from build123d import *

# Parameters (mm, degrees)
ESQUISSE1_W             = 24
ESQUISSE1_H             = 22
BOSS_EXTRU_1_DEPTH      = 2
ENL_V_MAT_EXTRU_1_DEPTH = 2
ESQUISSE3_R             = 1.75
ENL_V_MAT_EXTRU_2_DEPTH = 2
ESQUISSE4_R             = 2.894655209
ENL_V_MAT_EXTRU_3_DEPTH = 2
BOSS_EXTRU_2_DEPTH      = 10
ESQUISSE6_W             = 10
ESQUISSE6_H             = 10
ENL_V_MAT_EXTRU_4_DEPTH = 10
BOSS_EXTRU_3_DEPTH      = 2


with BuildPart() as part:
    # Esquisse1 → Boss.-Extru.1 (new body)
    with BuildSketch(Plane(origin=(0, 0, 0), x_dir=(1, 0, 0), z_dir=(0, 1, 0))):
        with Locations((12, 11)):
            Rectangle(ESQUISSE1_W, ESQUISSE1_H)
    extrude(amount=BOSS_EXTRU_1_DEPTH)

    # Esquisse2 → Enlèv. mat.-Extru.1 (cut)
    with BuildSketch(Plane(origin=(0, 2, 0), x_dir=(1, 0, 0), z_dir=(0, 1, 0))):
        Polygon((1, 21), (23, 21), (23, 10), (13, 10), (13, 1), (1, 1), align=None)
    extrude(amount=-ENL_V_MAT_EXTRU_1_DEPTH, mode=Mode.SUBTRACT)

    # Esquisse3 → Enlèv. mat.-Extru.2 (cut)
    with BuildSketch(Plane(origin=(0, 2, 0), x_dir=(1, 0, 0), z_dir=(0, 1, 0))):
        with Locations((18.75, 5)):
            Circle(ESQUISSE3_R)
    extrude(amount=-ENL_V_MAT_EXTRU_2_DEPTH, mode=Mode.SUBTRACT)

    # Esquisse4 → Enlèv. mat.-Extru.3 (cut)
    with BuildSketch(Plane(origin=(0, 2, 0), x_dir=(1, 0, 0), z_dir=(0, 1, 0))):
        with Locations((18.75, 5)):
            Circle(ESQUISSE4_R)
    extrude(amount=-ENL_V_MAT_EXTRU_3_DEPTH, mode=Mode.SUBTRACT)

    # Esquisse5 → Boss.-Extru.2 (add)
    with BuildSketch(Plane(origin=(0, 2, 0), x_dir=(1, 0, 0), z_dir=(0, 1, 0))):
        Polygon((14, 0), (14, 9), (24, 9), (24, 22), (0, 22), (0, 0), align=None)
        Polygon((1, 1), (1, 21), (23, 21), (23, 10), (13, 10), (13, 1), align=None, mode=Mode.SUBTRACT)
    extrude(amount=BOSS_EXTRU_2_DEPTH)

    # Esquisse6 → Enlèv. mat.-Extru.4 (cut)
    with BuildSketch(Plane.XY):
        with Locations((7, 5)):
            Rectangle(ESQUISSE6_W, ESQUISSE6_H)
    extrude(amount=-ENL_V_MAT_EXTRU_4_DEPTH, mode=Mode.SUBTRACT)

    # Esquisse8 → Boss.-Extru.3 (add)
    with BuildSketch(Plane(origin=(0, 12, 0), x_dir=(1, 0, 0), z_dir=(0, 1, 0))):
        Polygon((0, 0), (0, 22), (24, 22), (24, 9), (14, 9), (14, 0), align=None)
    extrude(amount=BOSS_EXTRU_3_DEPTH)


solid = part.part
The listing builds one solid part. Answer for the finished solid, in the listing's coordinates (mm). A direction names the side the tool comes from. Coordinates: 2 decimals unless noted, no trailing zeros. Order: outer loops, then holes, each group sorted by start corner. A loop starts at its lowest first (then second) coordinate and runs counter-clockwise, first axis right, second up.
Q1. A cutting plane is placed at D-D, the plane x = 18.75. Write down the section's boundary in (y, z), and give its area (3 significant figures).
Q2. Which of the six approach directions +Z, -Z, +X, -X, +Y, -Y give full straight-line access (tool end or side, diameter ignored) to faces 5 (the face through (6.9, 10, -0.5)), 6 (the face through (13, 6, -6)), 7 (the face through (19, 8, -9))?
Q3. A cutting plane is placed at C-C, the plane y = 6. Write down the section's boundary in (x, z).
Q4. A cutting plane is placed at B-B, the plane z = -4.25. Write down the section's boundary in (x, y), and give its area (3 significant figures).
Q5. Given P1, Ø2, axis at x = 19, z = -3.5, coming from the +Y side; P2, Ø10, axis at x = 20, z = -3, coming from the +Y side; P3, Ø0.5, axis at y = 5.5, z = -0.5, coming from the +X side; P4, Ø3.5, axis at x = 8.5, y = 5.5, coming from the +Z side, each flat-ended and moving along its own axis, determine where each tip first touches the part or whether it passes through.
Q6. Consider line 1 (Z direction, x = 18.75, y = 0.95); line 2 (X direction, y = 0.7, z = -5); line 3 (X direction, y = 6.25, z = -6.5). Determine where each line is inside the solid, lowest interval first.
Q7. A cutting plane is placed at A-A, the plane x = 6.25. Write down the section's boundary in (y, z), and give its area (3 significant figures).
Q8. For a pull along X with two mould halves and no side action, classify faces 1 (the face through (10, 14, -14)), 2 (the face through (14, 8, -5)), 3 (the face through (18.37, 1.01, -7.87)), 4 (the face through (0, 7, -11)) as pulls with the +X half, pulls with the -X half, needs draft (parallel to the pull), parting line crosses it, or undercut.
Answers follow:
1. outline: (0, -22) - (14, -22) - (14, -9) - (2, -9) - (2, -7.89) - (0, -7.89) - (0, -10) - (12, -10) - (12, -21) - (0, -21) - close; (0, -2.11) - (2, -2.11) - (2, 0) - (0, 0) - close
1. area: 56.4 mm2
2. face 5: +Z, -Y
2. face 6: -Y
2. face 7: +Z, +X, +Y
3. outline: (0, -22) - (24, -22) - (24, -9) - (14, -9) - (14, 0) - (12, 0) - (12, -1) - (13, -1) - (13, -10) - (23, -10) - (23, -21) - (1, -21) - (1, -1) - (2, -1) - (2, 0) - (0, 0) - close
4. outline: (0, 0) - (1, 0) - (1, 12) - (13, 12) - (13, 0) - (15.95, 0) - (15.95, 2) - (14, 2) - (14, 14) - (0, 14) - close; (21.55, 0) - (24, 0) - (24, 2) - (21.55, 2) - close
4. area: 60.8 mm2
5. P1: passes through
5. P2: stops at y = 2
5. P3: stops at x = 14
5. P4: stops at z = -21
6. line 1: z = -22 to -21, -10 to -7.89, -2.11 to 0
6. line 2: x = 0 to 1, 13 to 15.86, 21.64 to 24
6. line 3: x = 0 to 1, 13 to 14
7. outline: (0, -22) - (14, -22) - (14, 0) - (10, 0) - (10, -1) - (12, -1) - (12, -21) - (0, -21) - close
7. area: 58.0 mm2
8. face 1: needs draft
8. face 2: pulls with the +X half
8. face 3: undercut
8. face 4: pulls with the -X half
